from build123d import *

# Parameters (mm, degrees)
SKETCH1_R           = 1.6
BOSS_EXTRUDE1_DEPTH = 2


with BuildPart() as part:
    # Sketch1 → Boss-Extrude1 (new body)
    with BuildSketch(Plane.XY):
        with BuildLine():
            Line((-48.044206104, 75), (-48.044206104, -65))
            ThreePointArc((-48.044206104, -65), (-50.973138292, -72.071067812), (-58.044206104, -75))
            Line((-58.044206104, -75), (-68, -75))
            Line((-68, -75), (-68, -80))
            ThreePointArc((-68, -80), (-65.071067812, -87.071067812), (-58, -90))
            Line((-58, -90), (58, -90))
            ThreePointArc((58, -90), (65.071067812, -87.071067812), (68, -80))
            Line((68, -80), (68, -75))
            Line((68, -75), (57.867381689, -75))
            ThreePointArc((57.867381689, -75), (50.827572313, -72.08401548), (47.911587793, -65.044206104))
            Line((47.911587793, -65.044206104), (47.911587793, 75))
            ThreePointArc((47.911587793, 75), (44.955793896, 77.955793896), (42, 75))
            Line((42, 75), (42, -17))
            ThreePointArc((42, -17), (39.071067812, -24.071067812), (32, -27))
            Line((32, -27), (20.5, -27))
            ThreePointArc((20.5, -27), (17.5, -30), (20.5, -33))
            Line((20.5, -33), (32.044206104, -33))
            ThreePointArc((32.044206104, -33), (39.08401548, -35.91598452), (42, -42.955793896))
            Line((42, -42.955793896), (42, -65.044206104))
            ThreePointArc((42, -65.044206104), (39.08401548, -72.08401548), (32.044206104, -75))
            Line((32.044206104, -75), (32.044206104, -82.72))
            Line((32.044206104, -82.72), (-32.044206104, -82.72))
            Line((-32.044206104, -82.72), (-32.044206104, -75))
            ThreePointArc((-32.044206104, -75), (-39.115273915, -72.071067812), (-42.044206104, -65))
            Line((-42.044206104, -65), (-42.044206104, -43))
            ThreePointArc((-42.044206104, -43), (-39.115273915, -35.928932188), (-32.044206104, -33))
            Line((-32.044206104, -33), (-20, -33))
            ThreePointArc((-20, -33), (-17, -30), (-20, -27))
            Line((-20, -27), (-32.044206104, -27))
            ThreePointArc((-32.044206104, -27), (-39.115273915, -24.071067812), (-42.044206104, -17))
            Line((-42.044206104, -17), (-42.044206104, 75))
            ThreePointArc((-42.044206104, 75), (-45.044206104, 78), (-48.044206104, 75))
        make_face()
        with Locations((-45.044206104, 75)):
            Circle(SKETCH1_R, mode=Mode.SUBTRACT)
        with Locations((44.955793896, 75)):
            Circle(SKETCH1_R, mode=Mode.SUBTRACT)
        with Locations((-34.7, -80)):
            Circle(SKETCH1_R, mode=Mode.SUBTRACT)
        with Locations((34.7, -80)):
            Circle(SKETCH1_R, mode=Mode.SUBTRACT)
        with Locations((-20, -30)):
            Circle(SKETCH1_R, mode=Mode.SUBTRACT)
        with Locations((20.5, -30)):
            Circle(SKETCH1_R, mode=Mode.SUBTRACT)
    extrude(amount=BOSS_EXTRUDE1_DEPTH)


solid = part.part
Here's how the part is built. I have some questions about the finished solid (model axes, mm). A direction names the side the tool comes from. Round coordinates to 2 decimals unless told otherwise and drop trailing zeros. Loops run counter-clockwise (first coordinate to the right, second up) from the corner with the lowest first, then second, coordinate; pieces in that order, holes last. Notation, with made-up numbers: (67, -4) - (86, -4) arc R15 cw to (86, 7) - close; hole circle Ø5 at (85, 21). An arc over 180 degrees is marked (long way). One line per question, with ' | ' between items. Start each with the question number.
Q1. I want a section at C-C (x = 15). Write out the boundary of the cut face in (y, z).
Q2. I want a section at A-A (y = 35). Write out the boundary of the cut face in (x, z), then the cut area to 3 significant figures.
Q3. I want a section at D-D (x = -50). Write out the boundary of the cut face in (y, z).
Q4. I want a section at B-B (z = 0.4). State how many separate pieces and enclosed holes the cut face has, then the cut area to 3 significant figures.
Q5. Will these pins go through, and if not, where does the flat tip stop? pin 1 (1 mm diameter, centred on x = 63, z = 1, fed in from +Y); pin 2 (0.6 mm diameter, centred on y = -50.5, z = 1.5, fed in from -X); pin 3 (0.6 mm diameter, centred on x = 28, z = 1.5, fed in from +Y).
Q6. We'd pull the mould along Y, two halves only. Please class faces 1 (the cylindrical face through (50.905, -72.161, 0.986)), 2 (the cylindrical face through (39.16, -72.01, 0.99)), 3 (the cylindrical face through (-39.193, -36.007, 0.986)), 4 (the flat face through (-26, -30, 0)): +Y half, -Y half, draft (parallel to the pull), parting line (faces both ways), or undercut.
Q7. For faces 5 (the cylindrical face through (-39.037, -72.148, 0.986)), 6 (the cylindrical face through (-50.9, -72, 1)), 7 (the cylindrical face through (-39.037, -24.148, 0.986)), which set-ups out of +Z, -Z, +X, -X, +Y, -Y let a thin tool reach every point of the face, with its end or its side?
Q8. Please list where these lines run through material, in increasing order: line 1 (Y direction, x = 20.5, z = 1.35); line 2 (X direction, y = 75, z = 0.85); line 3 (X direction, y = 33, z = 0.75). Write a range as [from, to].
Response values:
1) outline: (-90, 0) - (-82.72, 0) - (-82.72, 2) - (-90, 2) - close
2) outline: (-48.04, 0) - (-42.04, 0) - (-42.04, 2) - (-48.04, 2) - close; (42, 0) - (47.91, 0) - (47.91, 2) - (42, 2) - close | area: 23.8 mm²
3) outline: (-90, 0) - (-70.94, 0) - (-70.94, 2) - (-90, 2) - close
4) separate pieces: 1 | enclosed holes: 6 | area: 3,730 mm²
5) pin 1: stops at y = -75 | pin 2: stops at x = -48.04 | pin 3: stops at y = -27
6) face 1: +Y half | face 2: undercut | face 3: undercut | face 4: draft
7) face 5: +Z, -Z | face 6: +Z, -Z, -X, +Y | face 7: +Z, -Z, +Y
8) line 1: y = [-90, -82.72], [-33, -31.6], [-28.4, -27] | line 2: x = [-48.04, -46.64], [-43.44, -42.04], [42, 43.36], [46.56, 47.91] | line 3: x = [-48.04, -42.04], [42, 47.91]
